Part model, mm, in its own coordinate system. A direction names the side the tool comes from. Round coordinates to 2 decimals unless told otherwise and drop trailing zeros. Loops run counter-clockwise (first coordinate to the right, second up) from the corner with the lowest first, then second, coordinate; pieces in that order, holes last.
1) Band-saw the part on C-C, the plane z = 689. Write the cut outline in (x, y).
2) Band-saw the part on D-D, the plane z = 50.8. Write the cut outline in (x, y) (3 decimals).
3) 3-axis set-ups, long thin cutter, end or side, ignore diameter. For faces 4 (the flat face through (-4, 4, 12.7)), 5 (the cylindrical face through (-1.74, -279.15, 64.02)), 6 (the flat face through (-4, 4, 0)): which of +Z, -Z, +X, -X, +Y, -Y reach the whole face in a straight line?
4) Band-saw the part on A-A, the plane y = 0. Write the cut outline in (x, z), then the cut area to 3 significant figures.
5) Band-saw the part on B-B, the plane x = -249.5. Write the cut outline in (y, z).
6) Drop flat-ended pins along their axis: P1, Ø8, axis at y = 104, z = 270, coming from the -X side; P2, Ø5, axis at y = 162.5, z = 485.5, coming from the -X side; P3, Ø2, axis at y = 177, z = 162.5, coming from the -X side. Give the stop position or say it passes through.
7) Probe line 1 (Y direction, x = 0, z = 303.5); line 2 (Z direction, x = 0, y = -278) (3 decimals); line 3 (Z direction, x = -139, y = 206.5). List the from-to ranges inside material, lowest first.
8) Mould opens along X. For faces 1 (the flat face through (147, -231, 762)), 2 (the cylindrical face through (-272.786, 12.005, 382.105)), 3 (the cylindrical face through (-285.474, 12.564, 375.666)) say: +X half, -X half, draft (parallel to the pull), parting line (faces both ways), or undercut.
from build123d import *

# Parameters (mm, degrees)
F0_R     = 285.75
F1_DEPTH = 762
F2_T     = -12.7
F3_R     = 13.335
F4_DEPTH = 327.66


with BuildPart() as f1:
    # F0 (on Top) → F1 (new body)
    with BuildSketch(Plane.XY):
        Circle(F0_R)
    extrude(amount=F1_DEPTH)

    # F2
    f2_openings = [f1.faces().sort_by_distance(p)[0] for p in [
        (0, 0, 762),
    ]]
    offset(amount=F2_T, openings=f2_openings)

    # F3 (on Front) → F4 (cut)
    with BuildSketch(Plane.XZ):
        with Locations((0, 50.8)):
            Circle(F3_R)
    extrude(amount=F4_DEPTH, mode=Mode.SUBTRACT)


solid = f1.part
Reported:
1. outline: circle Ø571.5 at (0, 0); hole circle Ø546.1 at (0, 0)
2. outline: (-13.335, -285.439) - (-13.335, -272.724) arc R273.05 cw (long way) to (13.335, -272.724) - (13.335, -285.439) arc R285.75 ccw (long way) to start
3. face 4: +Z
3. face 5: -Y
3. face 6: -Z, +X, -X, +Y, -Y
4. outline: (-285.75, 0) - (285.75, 0) - (285.75, 762) - (273.05, 762) - (273.05, 12.7) - (-273.05, 12.7) - (-273.05, 762) - (-285.75, 762) - close
4. area: 26,300 mm2
5. outline: (-139.29, 0) - (139.29, 0) - (139.29, 762) - (110.93, 762) - (110.93, 12.7) - (-110.93, 12.7) - (-110.93, 762) - (-139.29, 762) - close
6. P1: stops at x = -267.68
6. P2: stops at x = -236.76
6. P3: stops at x = -225.12
7. line 1: y = -285.75 to -273.05, 273.05 to 285.75
7. line 2: z = 0 to 37.465, 64.135 to 762
7. line 3: z = 0 to 12.7
8. face 1: draft
8. face 2: undercut
8. face 3: parting line
